```python
from build123d import *

# Parameters (mm, degrees)
SKETCH_1_R          = 1.65
SKETCH_1_R_2        = 5.5
EXTRUDE_1_DEPTH     = 2
SKETCH_2_R          = 1.65
CUT_EXTRUDE_2_DEPTH = 73.378330115
FILLET_1_R          = 2


with BuildPart() as part:
    # Эскиз1 → Бобышка-Вытянуть1 (new body)
    with BuildSketch(Plane(origin=(0, 0, 0), x_dir=(1, 0, 0), z_dir=(0, 1, 0))):
        with BuildLine():
            Line((-9.325751537, 7.551844693), (-20.594367979, 16.676990363))
            ThreePointArc((-20.594367979, 16.676990363), (-11.408544065, 23.918510035), (0, 26.5))
            ThreePointArc((0, 26.5), (9.472405203, 24.74921291), (17.693175332, 19.728191673))
            Line((17.693175332, 19.728191673), (40.060019619, -0.331452118))
            ThreePointArc((40.060019619, -0.331452118), (52.448537608, -15.858861968), (59.088465181, -34.580165246))
            ThreePointArc((59.088465181, -34.580165246), (54.221507729, -41.53090083), (47.270772145, -36.663943378))
            ThreePointArc((47.270772145, -36.663943378), (35.208034426, -12.373999402), (11.905757948, 1.500975575))
            ThreePointArc((11.905757948, 1.500975575), (-3.288975911, -11.540478216), (-9.325751537, 7.551844693))
        make_face()
        with Locations(Location((-6.322604321, 6.40505071, 0), (0, 0, 270))):
            Circle(SKETCH_1_R, mode=Mode.SUBTRACT)
        with Locations(Location((0, 0, 0), (0, 0, 270))):
            Circle(SKETCH_1_R_2, mode=Mode.SUBTRACT)
        with Locations(Location((8.708238788, 2.273010605, 0), (0, 0, 270))):
            Circle(SKETCH_1_R, mode=Mode.SUBTRACT)
        with Locations(Location((-2.385634467, -8.678061315, 0), (0, 0, 270))):
            Circle(SKETCH_1_R, mode=Mode.SUBTRACT)
    extrude(amount=EXTRUDE_1_DEPTH)

    # Эскиз2 → Вырез-Вытянуть2 (cut, through all)
    with BuildSketch(Plane(origin=(0, 2, 0), x_dir=(1, 0, 0), z_dir=(0, 1, 0))):
        with Locations(Location((-3.993908086, 22.650578319, 0), (0, 0, 270))):
            Circle(SKETCH_2_R)
        with Locations(Location((-13.192258036, 18.840497019, 0), (0, 0, 90))):
            Circle(SKETCH_2_R)
        with Locations(Location((46.765371804, -18, 0), (0, 0, 270))):
            Circle(SKETCH_2_R)
        with Locations(Location((53.179618663, -35.622998406, 0), (0, 0, 270))):
            Circle(SKETCH_2_R)
        with Locations(Location((34.710530923, -3.633600072, 0), (0, 0, 270))):
            Circle(SKETCH_2_R)
    extrude(amount=-CUT_EXTRUDE_2_DEPTH, mode=Mode.SUBTRACT)

    # Скругление1
    fillet_1_edges = [part.edges().sort_by_distance(p)[0] for p in [
        (11.905757948, 1, -1.500975575),
    ]]
    fillet(fillet_1_edges, radius=FILLET_1_R)


solid = part.part
```
Here's how the part is built. I have some questions about the finished solid (model axes, mm). Give positions to 0.01 mm unless a question says otherwise; leave off trailing zeros. Write each loop counter-clockwise with the first axis right and the second up, starting at its lowest first coordinate (ties: lowest second). Pieces come first, ordered by that corner, then holes.
(1) If I drill on L1, parallel to Z at x = -4.5, y = 1.85; L2, parallel to X at y = 0.7, z = -4; L3, parallel to X at y = 1.8, z = -23, over which ranges is the centre line in solid material (lowest first)?
Output values:
L1: z = -26.12 to -24.22, -21.08 to -3.16, 3.16 to 11.12
L2: x = -11.31 to -3.77, 3.77 to 35.23
L3: x = -13.16 to -5.61, -2.38 to 13.16
(2) Thinking about a two-plate mould opening in Z: for faces 1 (the face through (28.72, 0.99, -9.84)), 2 (the face through (36.371, 0.986, 13.676)), 3 (the face through (-3.39, 0.99, 7.37)), 4 (the face through (-14.88, 0.99, -12.05)), which applies, pulls with the +Z half, pulls with the -Z half, needs draft (parallel to the pull), parting line crosses it, or undercut?
Output values:
face 1: pulls with the -Z half
face 2: pulls with the +Z half
face 3: undercut
face 4: undercut
(3) Will these pins go through, and if not, where does the flat tip stop? pin 1 (4 mm diameter, centred on x = 34.71, z = 3.63, fed in from -Y); pin 2 (1 mm diameter, centred on y = 0.5, z = -3.5, fed in from +X).
Output values:
pin 1: stops at y = 0
pin 2: stops at x = 36.35
(4) Imagine slicing it at A-A, the plane x = 3. Write out the boundary of the cut face in (y, z).
Output values:
outline: (0, -26.33) - (2, -26.33) - (2, -4.61) - (0, -4.61) - close; (0, 4.61) - (2, 4.61) - (2, 11.62) - (0, 11.62) - close
(5) Imagine slicing it at C-C, the plane y = 0.5. Count the separate pieces of the cut face and the enclosed holes in it, and give its area (3 significant figures).
Output values:
separate pieces: 1
enclosed holes: 9
area: 1,660 mm2
(6) Imagine slicing it at B-B, the plane z = 18. Write out the boundary of the cut face in (x, y).
Output values:
outline: (39.69, 0) - (45.12, 0) - (45.12, 2) - (39.69, 2) - close; (48.42, 0) - (53.58, 0) - (53.58, 2) - (48.42, 2) - close
